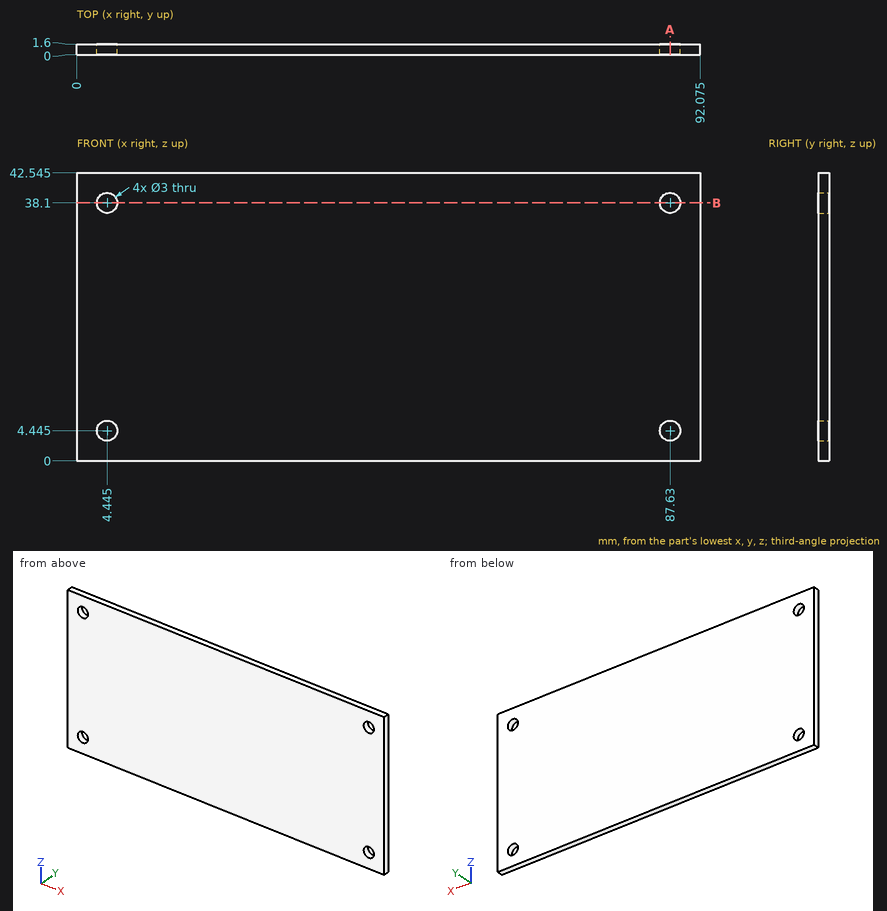
Geometry: see drawing. Coordinates: mm, zero at the bounding-box minimum. Coordinates: 2 decimals unless noted, no trailing zeros. Loops run counter-clockwise (first coordinate to the right, second up) from the corner with the lowest first, then second, coordinate; pieces in that order, holes last. Notation, with made-up numbers: M 79,61 L 123,61 A13 ccw 123,69 Z; hole C -16,63.5 d8. An arc over 180 degrees is marked long. Answer in a Markdown table with one row per item.
Q1. Section B-B on z = 38.1. Return the cut outline in (x, y) (3 decimals).
Answers below:
| item | result |
|---|---|
| outline | M 0,0 L 2.945,0 L 2.945,1.6 L 0,1.6 Z; M 5.945,0 L 86.13,0 L 86.13,1.6 L 5.945,1.6 Z; M 89.13,0 L 92.075,0 L 92.075,1.6 L 89.13,1.6 Z |
Q2. Section A-A on x = 87.63. Return the cut outline in (y, z) (3 decimals), plus the area to 3 significant figures.
Answers below:
| item | result |
|---|---|
| outline | M 0,0 L 1.6,0 L 1.6,2.945 L 0,2.945 Z; M 0,5.945 L 1.6,5.945 L 1.6,36.6 L 0,36.6 Z; M 0,39.6 L 1.6,39.6 L 1.6,42.545 L 0,42.545 Z |
| area | 58.5 mm^2 |
Q3. Ray query, probe 1 along X at (y, z) = (1, 38) (3 decimals); probe 2 along Z at (x, y) = (88.5, 1.25) (3 decimals); probe 3 along X at (y, z) = (1.5, 5.5) (3 decimals). Return the intervals inside material, ascending. Write a range as from..to.
Answers below:
| item | result |
|---|---|
| probe 1 | x = 0..2.948, 5.942..86.133, 89.127..92.075 |
| probe 2 | z = 0..3.223, 5.667..36.878, 39.322..42.545 |
| probe 3 | x = 0..3.379, 5.511..86.564, 88.696..92.075 |
